The model under review builds one solid part; all positions refer to its coordinate system, in mm. A direction names the side the tool comes from. Give positions to 0.01 mm unless a question says otherwise; leave off trailing zeros. Loops run counter-clockwise (first coordinate to the right, second up) from the corner with the lowest first, then second, coordinate; pieces in that order, holes last. Notation, with made-up numbers: (67.5, -12.75) -> (89.5, -12.75) arc R21 ccw to (89.5, 14.25) -> close; hole circle Ø8 at (-33.75, 75.5). An arc over 180 degrees is marked (long way). Write each question's results on one line, items separated by ' | '. Start each with the question number.
Q1. We need section C-C (z = 30). Give the number of separate pieces and of enclosed holes in the cut face, plus the area to 3 significant figures.
Q2. We need section B-B (z = 60). Write out the cut boundary in (x, y), plus the area to 3 significant figures.
Q3. Insertion check: pin 1 Ø4 at (y, z) = (461.5, 111.5) entering from +X; pin 2 Ø10 at (y, z) = (444.5, 90) entering from +X; pin 3 Ø10 at (x, z) = (420, 70.5) entering from -Y; pin 4 Ø7 at (y, z) = (394.5, 90) entering from +X. Each pin has a flat end and moves straight along its axis. Give the tip position at first contact, or say it passes through.
Q4. Wall thickness on L1, parallel to Z at x = 394.5, y = 444.5; L2, parallel to Z at x = 411, y = 394; L3, parallel to Y at x = 442.5, z = 32.5: over which ranges is each line inside the solid? List them lowest first. Write a range as [from, to].
Q5. Mouldability with a two-part tool opening along Y and no side actions: class faces 4 (the face through (431.95, 561, 140)), 5 (the face through (457.2, 473, 88)), 6 (the face through (419.633, 560.237, 4.811)) as released by +Y, released by -Y, zero draft, split by the parting line, or undercut.
Q6. Machinability: for faces 1 (the face through (425.45, 520, 97)), 2 (the face through (428.45, 560, 140)), 3 (the face through (441, 561, 135)), which of the approach directions +Z, -Z, +X, -X, +Y, -Y give a long, thin tool a straight path to every point of the face, cutting with its end or side? Answer none if there is none.
Q7. We need section A-A (y = 394.5). Write out the cut boundary in (x, z), plus the area to 3 significant figures.
Q8. We need section D-D (x = 415.5). Write out the cut boundary in (y, z), plus the area to 3 significant figures.
from build123d import *

# Parameters (mm, degrees)
BOSS_EXTRUDE1_DEPTH = 120
SKETCH3_R           = 4.25
CUT_EXTRUDE1_DEPTH  = 120
SKETCH5_R           = 10
CUT_EXTRUDE2_DEPTH  = 53
SKETCH6_R           = 4.25
CUT_EXTRUDE3_DEPTH  = 103
SKETCH7_W           = 76.2
SKETCH7_H           = 120
BOSS_EXTRUDE2_DEPTH = 101.6
SKETCH8_R           = 41.35
CUT_EXTRUDE4_DEPTH  = 31.75
CUT_EXTRUDE5_START  = -31.75
SKETCH9_R           = 41.35
CUT_EXTRUDE5_DEPTH  = 31.75
SKETCH10_R          = 38.1
CUT_EXTRUDE6_DEPTH  = 76.2
SKETCH13_W          = 76.2
SKETCH13_H          = 120
BOSS_EXTRUDE3_DEPTH = 6
CUT_EXTRUDE7_DEPTH  = 84.4
SKETCH12_R          = 6.25
CUT_EXTRUDE8_DEPTH  = 5.5
FILLET1_R           = 16
SKETCH18_W          = 32
SKETCH18_H          = 10
BOSS_EXTRUDE6_DEPTH = 15
BOSS_EXTRUDE7_DEPTH = 10
FILLET3_R           = 5


with BuildPart() as part:
    # Sketch1 → Boss-Extrude1 (new body)
    with BuildSketch(Plane.XY):
        Polygon((381, 457.2), (457.2, 457.2), (457.2, 431.8), (381, 357.2), align=None)
    extrude(amount=BOSS_EXTRUDE1_DEPTH)

    # Sketch3 → Cut-Extrude1 (cut)
    with BuildSketch(Plane(origin=(457.2, 0, 0), x_dir=(0, 0, -1), z_dir=(1, 0, 0))):
        with Locations(Location((-90, 394.5, 0), (0, 0, 90))):
            Circle(SKETCH3_R)
        with Locations(Location((-30, 394.5, 0), (0, 0, 90))):
            Circle(SKETCH3_R)
    extrude(amount=-CUT_EXTRUDE1_DEPTH, mode=Mode.SUBTRACT)

    # Sketch5 → Cut-Extrude2 (cut)
    with BuildSketch(Plane(origin=(457.2, 0, 0), x_dir=(0, 0, -1), z_dir=(1, 0, 0))):
        with Locations(Location((-90, 394.5, 0), (0, 0, 90))):
            Circle(SKETCH5_R)
        with Locations(Location((-30, 394.5, 0), (0, 0, 90))):
            Circle(SKETCH5_R)
        with Locations(Location((-90, 444.5, 0), (0, 0, 90))):
            Circle(SKETCH5_R)
        with Locations(Location((-30, 444.5, 0), (0, 0, 90))):
            Circle(SKETCH5_R)
    extrude(amount=-CUT_EXTRUDE2_DEPTH, mode=Mode.SUBTRACT)

    # Sketch6 → Cut-Extrude3 (cut)
    with BuildSketch(Plane(origin=(457.2, 0, 0), x_dir=(0, 0, -1), z_dir=(1, 0, 0))):
        with Locations(Location((-90, 444.5, 0), (0, 0, 90))):
            Circle(SKETCH6_R)
        with Locations(Location((-30, 444.5, 0), (0, 0, 90))):
            Circle(SKETCH6_R)
    extrude(amount=-CUT_EXTRUDE3_DEPTH, mode=Mode.SUBTRACT)

    # Sketch7 → Boss-Extrude2 (add)
    with BuildSketch(Plane(origin=(0, 457.2, 0), x_dir=(1, 0, 0), z_dir=(0, 1, 0))):
        with Locations((419.1, -60)):
            Rectangle(SKETCH7_W, SKETCH7_H)
    extrude(amount=BOSS_EXTRUDE2_DEPTH)

    # Sketch8 → Cut-Extrude4 (cut)
    with BuildSketch(Plane.ZY.offset(-381)):
        with Locations((60, 508)):
            Circle(SKETCH8_R)
    extrude(amount=-CUT_EXTRUDE4_DEPTH, mode=Mode.SUBTRACT)

    # Sketch9 → Cut-Extrude5 (cut)
    with BuildSketch(Plane(origin=(457.2, 0, 0), x_dir=(0, 0, -1), z_dir=(1, 0, 0)).offset(CUT_EXTRUDE5_START)):
        with Locations(Location((-60, 508, 0), (0, 0, 180))):
            Circle(SKETCH9_R)
    extrude(amount=CUT_EXTRUDE5_DEPTH, mode=Mode.SUBTRACT)

    # Sketch10 → Cut-Extrude6 (cut)
    with BuildSketch(Plane(origin=(457.2, 0, 0), x_dir=(0, 0, -1), z_dir=(1, 0, 0))):
        with Locations(Location((-60, 508, 0), (0, 0, 90))):
            Circle(SKETCH10_R)
    extrude(amount=-CUT_EXTRUDE6_DEPTH, mode=Mode.SUBTRACT)

    # Sketch13 → Boss-Extrude3 (add)
    with BuildSketch(Plane(origin=(0, 558.8, 0), x_dir=(1, 0, 0), z_dir=(0, 1, 0))):
        with Locations((419.1, -60)):
            Rectangle(SKETCH13_W, SKETCH13_H)
    extrude(amount=BOSS_EXTRUDE3_DEPTH)

    # Sketch11 → Cut-Extrude7 (cut)
    with BuildSketch(Plane(origin=(457.2, 0, 0), x_dir=(0, 0, -1), z_dir=(1, 0, 0))):
        with BuildLine():
            Line((-110, 550.25), (-110, 553))
            Line((-110, 553), (-107.25, 553))
            ThreePointArc((-107.25, 553), (-111.944543648, 554.944543648), (-110, 550.25))
        make_face()
        with BuildLine():
            Line((-107.25, 553), (-110, 553))
            Line((-110, 553), (-110, 550.25))
            ThreePointArc((-110, 550.25), (-108.055456352, 551.055456352), (-107.25, 553))
        make_face()
        with BuildLine():
            ThreePointArc((-7.25, 553), (-10, 555.75), (-12.75, 553))
            Line((-12.75, 553), (-10, 553))
            Line((-10, 553), (-10, 550.25))
            ThreePointArc((-10, 550.25), (-8.055456352, 551.055456352), (-7.25, 553))
        make_face()
        with BuildLine():
            Line((-10, 553), (-12.75, 553))
            ThreePointArc((-12.75, 553), (-11.944543648, 551.055456352), (-10, 550.25))
            Line((-10, 550.25), (-10, 553))
        make_face()
        with BuildLine():
            ThreePointArc((-7.25, 463), (-8.055456352, 464.944543648), (-10, 465.75))
            Line((-10, 465.75), (-10, 463))
            Line((-10, 463), (-12.75, 463))
            ThreePointArc((-12.75, 463), (-10, 460.25), (-7.25, 463))
        make_face()
        with BuildLine():
            Line((-10, 463), (-10, 465.75))
            ThreePointArc((-10, 465.75), (-11.944543648, 464.944543648), (-12.75, 463))
            Line((-12.75, 463), (-10, 463))
        make_face()
        with BuildLine():
            ThreePointArc((-107.25, 463), (-108.055456352, 464.944543648), (-110, 465.75))
            Line((-110, 465.75), (-110, 463))
            Line((-110, 463), (-107.25, 463))
        make_face()
        with BuildLine():
            Line((-110, 463), (-110, 465.75))
            ThreePointArc((-110, 465.75), (-111.944543648, 461.055456352), (-107.25, 463))
            Line((-107.25, 463), (-110, 463))
        make_face()
    extrude(amount=-CUT_EXTRUDE7_DEPTH, mode=Mode.SUBTRACT)

    # Sketch12 → Cut-Extrude8 (cut)
    with BuildSketch(Plane(origin=(457.2, 0, 0), x_dir=(0, 0, -1), z_dir=(1, 0, 0))):
        with Locations((-110, 553)):
            Circle(SKETCH12_R)
        with Locations((-10, 553)):
            Circle(SKETCH12_R)
        with Locations((-10, 463)):
            Circle(SKETCH12_R)
        with Locations((-110, 463)):
            Circle(SKETCH12_R)
    extrude(amount=-CUT_EXTRUDE8_DEPTH, mode=Mode.SUBTRACT)

    # Fillet1
    fillet1_edges = [part.edges().sort_by_distance(p)[0] for p in [
        (419.1, 564.8, 120),
        (419.1, 564.8, 0),
    ]]
    fillet(fillet1_edges, radius=FILLET1_R)

    # Sketch18 → Boss-Extrude6 (add)
    with BuildSketch(Plane.XY.offset(120)):
        with Locations((441.2, 527.8)):
            Rectangle(SKETCH18_W, SKETCH18_H)
    extrude(amount=BOSS_EXTRUDE6_DEPTH)

    # Sketch20 → Boss-Extrude7 (add)
    with BuildSketch(Plane.XY.offset(135)):
        Polygon((425.2, 588.682542047), (425.2, 532.8), (425.2, 522.8), (457.2, 522.8), (457.2, 536.682542047), (457.2, 588.682542047), align=None)
        with BuildLine():
            ThreePointArc((428.45, 584.682542047), (430.2, 586.432542047), (431.95, 584.682542047))
            Line((431.95, 584.682542047), (431.95, 536.8))
            ThreePointArc((431.95, 536.8), (430.2, 535.05), (428.45, 536.8))
            Line((428.45, 536.8), (428.45, 584.682542047))
        make_face(mode=Mode.SUBTRACT)
        with BuildLine():
            Line((450.45, 536.8), (450.45, 584.682542047))
            ThreePointArc((450.45, 584.682542047), (452.2, 586.432542047), (453.95, 584.682542047))
            Line((453.95, 584.682542047), (453.95, 536.8))
            ThreePointArc((453.95, 536.8), (452.2, 535.05), (450.45, 536.8))
        make_face(mode=Mode.SUBTRACT)
    extrude(amount=BOSS_EXTRUDE7_DEPTH)

    # Fillet3
    fillet3_edges = [part.edges().sort_by_distance(p)[0] for p in [
        (441.2, 522.8, 120),
        (425.2, 588.682542047, 140),
        (457.2, 588.682542047, 140),
        (441.2, 522.8, 145),
    ]]
    fillet(fillet3_edges, radius=FILLET3_R)


solid = part.part
Output:
1) separate pieces: 4 | enclosed holes: 0 | area: 7,010 mm2
2) outline: (381, 357.2) -> (457.2, 431.8) -> (457.2, 466.65) -> (425.45, 466.65) -> (425.45, 469.9) -> (412.75, 469.9) -> (412.75, 466.65) -> (381, 466.65) -> close; (381, 549.35) -> (412.75, 549.35) -> (412.75, 546.1) -> (425.45, 546.1) -> (425.45, 549.35) -> (457.2, 549.35) -> (457.2, 564.8) -> (381, 564.8) -> close | area: 6,760 mm2
3) pin 1: x = 451.7 | pin 2: x = 404.2 | pin 3: y = 390.49 | pin 4: through
4) L1: [0, 25.75], [34.25, 85.75], [94.25, 120] | L2: [0, 20.01], [39.99, 80.01], [99.99, 120] | L3: [417.41, 434.82], [454.18, 477.12], [538.88, 564.8]
5) face 4: undercut | face 5: zero draft | face 6: released by +Y
6) face 1: +X | face 2: +Z | face 3: +X, -X, +Y
7) outline: (381, 0) -> (419.1, 0) -> (419.1, 20) -> (404.2, 20) -> (404.2, 25.75) -> (381, 25.75) -> close; (381, 34.25) -> (404.2, 34.25) -> (404.2, 40) -> (419.1, 40) -> (419.1, 80) -> (404.2, 80) -> (404.2, 85.75) -> (381, 85.75) -> close; (381, 94.25) -> (404.2, 94.25) -> (404.2, 100) -> (419.1, 100) -> (419.1, 120) -> (381, 120) -> close | area: 3,580 mm2
8) outline: (390.98, 0) -> (548.8, 0) arc R16 ccw to (564.8, 16) -> (564.8, 104) arc R16 ccw to (548.8, 120) -> (390.98, 120) -> (390.98, 99.36) arc R10 cw (long way) to (390.98, 80.64) -> (390.98, 39.36) arc R10 cw (long way) to (390.98, 20.64) -> close; hole circle Ø20 at (444.5, 30); hole circle Ø20 at (444.5, 90); hole circle Ø5.5 at (463, 10); hole circle Ø5.5 at (463, 110); hole circle Ø76.2 at (508, 60); hole circle Ø5.5 at (553, 10); hole circle Ø5.5 at (553, 110) | area: 15,000 mm2
